Source: three-view drawing plus pictorial views. Frame: mm from the lowest corner of the part. A direction names the side the tool comes from. Coordinates: 2 decimals unless noted, no trailing zeros. Write each loop counter-clockwise with the first axis right and the second up, starting at its lowest first coordinate (ties: lowest second). Pieces come first, ordered by that corner, then holes. Notation, with made-up numbers: M 60,8 L 104,8 A19 ccw 104,19 Z; hole C 70,33 d5. An arc over 180 degrees is marked long. Use CSV: the item, a comma, the result in double quotes.
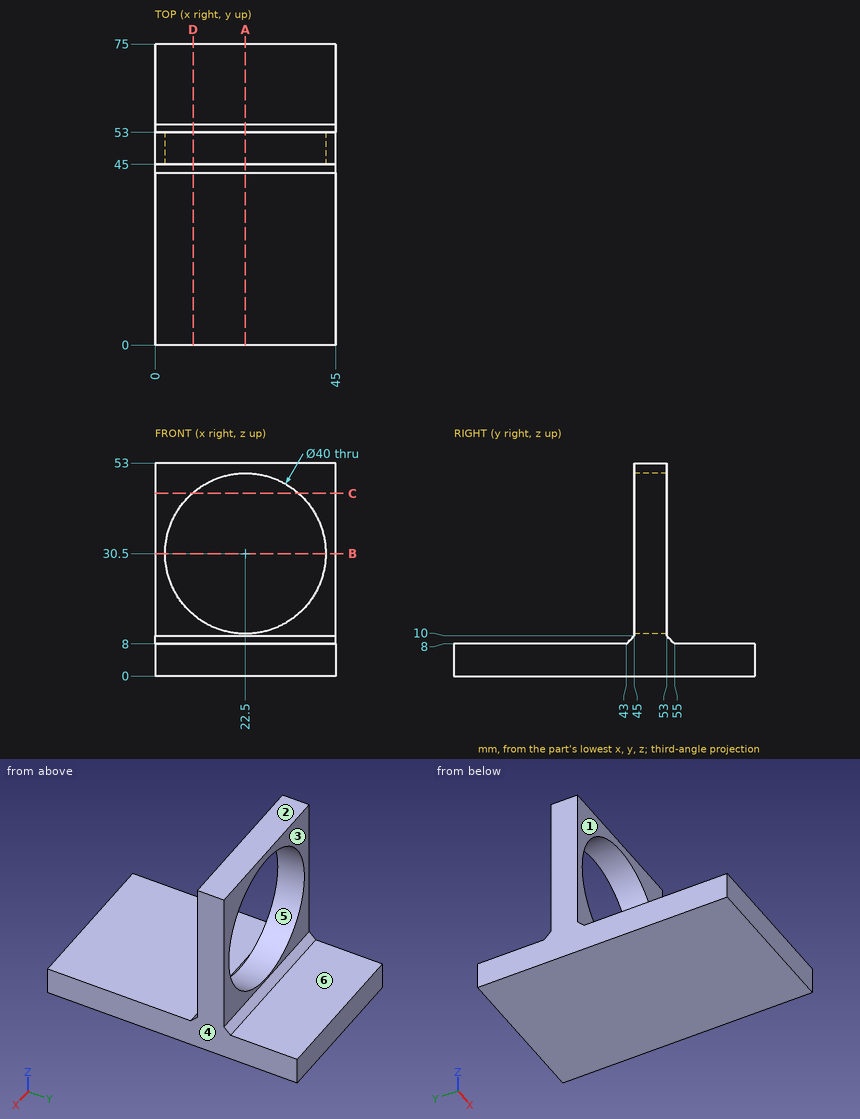
1. Section D-D (x = 9.5). Return loops of the section in (y, z), then the cut area to 3 significant figures.
Resolved:
outline,"M 0,0 L 75,0 L 75,8 L 55,8 L 53,10 L 53,15.3 L 45,15.3 L 45,10 L 43,8 L 0,8 Z; M 45,45.7 L 53,45.7 L 53,53 L 45,53 Z"
area,"721 mm^2"
2. Section C-C (z = 45.5). Return loops of the section in (x, y).
Resolved:
outline,"M 0,45 L 9.27,45 L 9.27,53 L 0,53 Z; M 35.73,45 L 45,45 L 45,53 L 35.73,53 Z"
3. Section A-A (x = 22.5). Return loops of the section in (y, z).
Resolved:
outline,"M 0,0 L 75,0 L 75,8 L 55,8 L 53,10 L 53,10.5 L 45,10.5 L 45,10 L 43,8 L 0,8 Z; M 45,50.5 L 53,50.5 L 53,53 L 45,53 Z"
4. Material intervals for line 1 (Z direction, x = 22.5, y = 50); line 2 (X direction, y = 49, z = 30); line 3 (Y direction, x = 9.5, z = 46), sorted ascending. Write a range as [from, to].
Resolved:
line 1,"z = [0, 10.5], [50.5, 53]"
line 2,"x = [0, 2.51], [42.49, 45]"
line 3,"y = [45, 53]"
5. Contact query for flat-ended pins moving along their axis: pin 1 Ø8 at (x, z) = (28.5, 45.5) entering from -Y; pin 2 Ø10 at (x, y) = (26, 63.5) entering from +Z; pin 3 Ø24 at (x, z) = (22.5, 30.5) entering from -Y; pin 4 Ø1.5 at (x, z) = (38.5, 18) entering from +Y. Output: stop coordinate, or through.
Resolved:
pin 1,"stops at y = 45"
pin 2,"stops at z = 8"
pin 3,"passes through"
pin 4,"stops at y = 53"
6. Access query for the marked faces 1, 2 and 3. Directions: +Z, -Z, +X, -X, +Y, -Y. A direction counts if a zero-diameter tool reaches every point of the face in a straight line with its end or side. Return the directions, or none.
Resolved:
face 1,"+Z, +X, -X, -Y"
face 2,"+Z, +X, -X, +Y, -Y"
face 3,"+Z, +X, -X, +Y"
7. Section B-B (z = 30.5). Return loops of the section in (x, y).
Resolved:
outline,"M 0,45 L 2.5,45 L 2.5,53 L 0,53 Z; M 42.5,45 L 45,45 L 45,53 L 42.5,53 Z"
8. Mould query, pull axis X, two halves, no side actions, for the marked faces 4, 5 and 6. Classes: pulls with the +X half, pulls with the -X half, needs draft (parallel to the pull), parting line crosses it, or undercut.
Resolved:
face 4,"pulls with the +X half"
face 5,"undercut"
face 6,"needs draft"
